from build123d import *

# Parameters (mm, degrees)
F0_R     = 42.229766
F1_DEPTH = 25
F3_DEPTH = 10
F4_R     = 12.738084
F5_DEPTH = 100


with BuildPart() as f1:
    # F0 (on Front) → F1 (new body)
    with BuildSketch(Plane.XZ):
        Circle(F0_R)
    extrude(amount=F1_DEPTH)

    # F2 (on Front) → F3 (cut)
    with BuildSketch(Plane.XZ):
        Polygon((0.760662, -14.179654), (12.660271, -6.431074), (11.899609, 7.74858), (-0.760662, 14.179654), (-12.660271, 6.431074), (-11.899609, -7.74858), align=None)
    extrude(amount=F3_DEPTH, mode=Mode.SUBTRACT)

    # F4 (on Front) → F5 (join)
    with BuildSketch(Plane.XZ):
        Circle(F4_R)
    extrude(amount=F5_DEPTH)


solid = f1.part
Design review of the part built by this model. Coordinates are the model's own, in mm. A direction names the side the tool comes from. Round coordinates to 2 decimals unless told otherwise and drop trailing zeros. Write each loop counter-clockwise with the first axis right and the second up, starting at its lowest first coordinate (ties: lowest second). Pieces come first, ordered by that corner, then holes. Notation, with made-up numbers: (33.25, -12.75) - (81.25, -12.75) arc R13 ccw to (81.25, 4.25) - close; hole circle Ø4 at (41.5, 86). An arc over 180 degrees is marked (long way). Return JSON: item names as keys, results as strings. Group by question number.
Item 1: We need section D-D on y = -11.5. Write out the cut boundary in (x, z).
Item 2: The part is to be moulded in two halves that separate along Z. For faces 1 (the face through (12.15, -61.98, 3.83)), 2 (the face through (0.95, -4.93, 13.31)), 3 (the face through (2.322, -4.93, -13.163)), 4 (the face through (0, -100, 0)), say which applies: pulls with the +Z half, pulls with the -Z half, needs draft (parallel to the pull), parting line crosses it, or undercut.
Item 3: We need section B-B on y = -80.5. Write out the cut boundary in (x, z), and give its area (3 significant figures).
Item 4: We need section A-A on z = 0. Write out the cut boundary in (x, y).
Item 5: We need section C-C on x = -21. Write out the cut boundary in (y, z), and give its area (3 significant figures).
Item 6: Insertion check: P1, Ø12, axis at x = -33.5, y = -27.5, coming from the -Z side; P2, Ø4, axis at x = 10, y = -24, coming from the +Z side; P3, Ø10, axis at y = -23, z = 10, coming from the -X side. Each pin has a flat end and moves straight along its axis. Give the tip position at first contact, or say it passes through.
Item 7: Machinability: for faces 5 (the face through (-1, 0, 1)), 6 (the face through (-12, -10, 6)), which of the approach directions +Z, -Z, +X, -X, +Y, -Y give a long, thin tool a straight path to every point of the face, cutting with its end or side? Answer none if there is none.
Item 8: For probe 1 along Z at (x, y) = (4.5, -31); probe 2 along Y at (x, z) = (12, -23); probe 3 along Z at (x, y) = (-0.5, -30), list the stretches that pass through material, from the lowest coordinate up. Write a range as [from, to].
Model answer:
{
 "1": {"outline": "circle Ø84.46 at (0, 0)"},
 "2": {"face 1": "parting line crosses it", "face 2": "undercut", "face 3": "undercut", "face 4": "needs draft"},
 "3": {"outline": "circle Ø25.48 at (0, 0)", "area": "510 mm²"},
 "4": {"outline": "(-42.23, -25) - (-12.74, -25) - (-12.74, -100) - (12.74, -100) - (12.74, -25) - (42.23, -25) - (42.23, 0) - (-42.23, 0) - close"},
 "5": {"outline": "(-25, -36.64) - (0, -36.64) - (0, 36.64) - (-25, 36.64) - close", "area": "1,830 mm²"},
 "6": {"P1": "stops at z = -31.57", "P2": "stops at z = 41.47", "P3": "stops at x = -41.93"},
 "7": {"face 5": "+Z, -Z, +X, -X, +Y", "face 6": "+Y"},
 "8": {"probe 1": "z = [-11.92, 11.92]", "probe 2": "y = [-25, 0]", "probe 3": "z = [-12.73, 12.73]"}
}
